```python
from build123d import *

# Parameters (mm, degrees)
SKETCH1_R               = 150
BOSS_EXTRUDE1_DEPTH     = 9.09
SKETCH2_R               = 146.82
CUT_EXTRUDE1_DEPTH      = 15
SKETCH5_R               = 90
BOSS_EXTRUDE2_DEPTH     = 15
CHAMFER1_SIZE           = 5
FILLET6_R               = 10
SKETCH6_R               = 1.55
CUT_EXTRUDE2_DEPTH      = 5
SKETCH7_R               = 16
CUT_EXTRUDE3_DEPTH      = 4.8
BOSS_EXTRUDE3_START     = 4.8
BOSS_EXTRUDE3_DEPTH     = 4.8
CIRPATTERN1_COUNT       = 30
SKETCH17_W              = 2.73
SKETCH17_H              = 90
SKETCH23_W              = 41
SKETCH23_H              = 20
CUT_EXTRUDE6_DEPTH      = 213.486594636
CUT_EXTRUDE7_DEPTH      = 213.486594636
CUT_EXTRUDE7_DEPTH_BACK = 213.486594636
SKETCH24_R              = 1.47
SKETCH26_R              = 150
SKETCH26_R_2            = 120
BOSS_EXTRUDE4_DEPTH     = 16.64


with BuildPart() as part:
    # Sketch1 → Boss-Extrude1 (new, symmetric)
    with BuildSketch(Plane.XY):
        Circle(SKETCH1_R)
    extrude(amount=BOSS_EXTRUDE1_DEPTH, both=True)

    # Sketch2 → Cut-Extrude1 (cut)
    with BuildSketch(Plane.XY.offset(9.09)):
        Circle(SKETCH2_R)
    extrude(amount=-CUT_EXTRUDE1_DEPTH, mode=Mode.SUBTRACT)

    # Sketch5 → Boss-Extrude2 (add)
    with BuildSketch(Plane.XY.offset(-5.91)):
        Circle(SKETCH5_R)
    extrude(amount=BOSS_EXTRUDE2_DEPTH)

    # Chamfer1
    chamfer1_edges = [part.edges().sort_by_distance(p)[0] for p in [
        (-90, 0, -5.91),
    ]]
    chamfer(chamfer1_edges, length=CHAMFER1_SIZE)

    # Fillet6
    fillet6_edges = [part.edges().sort_by_distance(p)[0] for p in [
        (-95, 0, -5.91),
    ]]
    fillet(fillet6_edges, radius=FILLET6_R)

    # Sketch6 → Cut-Extrude2 (cut)
    with BuildSketch(Plane.XY.offset(9.09)):
        with Locations((64.65, 0)):
            Circle(SKETCH6_R)
        with Locations((-68.33, 0)):
            Circle(SKETCH6_R)
        with Locations((-54.47, 24.14)):
            Circle(SKETCH6_R)
        with Locations((-54.47, -24.14)):
            Circle(SKETCH6_R)
        with Locations((50.79, -24.14)):
            Circle(SKETCH6_R)
        with Locations((50.79, 24.14)):
            Circle(SKETCH6_R)
    extrude(amount=-CUT_EXTRUDE2_DEPTH, mode=Mode.SUBTRACT)

    # Sketch7 → Cut-Extrude3 (cut)
    with BuildSketch(Plane.XY.offset(9.09)):
        Circle(SKETCH7_R)
    extrude(amount=-CUT_EXTRUDE3_DEPTH, mode=Mode.SUBTRACT)

    # Sketch8 → Boss-Extrude3 (add)
    with BuildSketch(Plane.XY.offset(4.29).offset(BOSS_EXTRUDE3_START)):
        with BuildLine():
            ThreePointArc((1.300521762, 15.947057507), (0.787845605, 15.007972717), (0.45011023, 13.992762443))
            ThreePointArc((0.45011023, 13.992762443), (0, 14), (-0.45011023, 13.992762443))
            ThreePointArc((-0.45011023, 13.992762443), (-0.787845605, 15.007972717), (-1.300521762, 15.947057507))
            ThreePointArc((-1.300521762, 15.947057507), (0, 16), (1.300521762, 15.947057507))
        make_face()
    boss_extrude3 = extrude(amount=-BOSS_EXTRUDE3_DEPTH)

    # CirPattern1: Boss-Extrude3 ×30 about axis
    cirpattern1_axis = Axis((0, 0, 0), (0, 0, 1))
    for i in range(1, CIRPATTERN1_COUNT):
        add(boss_extrude3.rotate(cirpattern1_axis, i * 360 / CIRPATTERN1_COUNT))

    # Sketch17 → Cut-Revolve4 (revolve, cut)
    with BuildSketch(Plane(origin=(0, 0, 0), x_dir=(0, 0, -1), z_dir=(1, 0, 0))):
        with Locations((-4.545, 45)):
            Rectangle(SKETCH17_W, SKETCH17_H)
    revolve(axis=Axis((0, 0, -0.91), (0, 0, 1)), mode=Mode.SUBTRACT)


with BuildPart() as cut_revolve4_piece_1:
    # of the separate pieces the step leaves, piece 1, a body of its own (cut_revolve4_pieces)
    add(part.part.solids().sort_by_distance((99.142135624, 0, -5.91))[0])

    # Sketch23 → Cut-Extrude6 (cut, through all)
    with BuildSketch(Plane.XY.offset(3.18)):
        with Locations((-10.44, 0)):
            Rectangle(SKETCH23_W, SKETCH23_H)
    extrude(amount=-CUT_EXTRUDE6_DEPTH, mode=Mode.SUBTRACT)

    # Sketch24 → Cut-Extrude7 (cut, two sides: drawn at the far end of the back side and taken through both)
    with BuildSketch(Plane.XY.offset(3.18).offset(-CUT_EXTRUDE7_DEPTH_BACK)):
        with Locations((-35.419501393, -5.08)):
            Circle(SKETCH24_R)
        with Locations((14.680498607, -5.08)):
            Circle(SKETCH24_R)
        with Locations((-35.419501393, 5.08)):
            Circle(SKETCH24_R)
        with Locations((14.680498607, 5.08)):
            Circle(SKETCH24_R)
    extrude(amount=CUT_EXTRUDE7_DEPTH + CUT_EXTRUDE7_DEPTH_BACK, mode=Mode.SUBTRACT)

    # Sketch26 → Boss-Extrude4 (add)
    with BuildSketch(Plane(origin=(0, 0, -9.09), x_dir=(-1, 0, 0), z_dir=(0, 0, -1))):
        Circle(SKETCH26_R)
        Circle(SKETCH26_R_2, mode=Mode.SUBTRACT)
    extrude(amount=BOSS_EXTRUDE4_DEPTH)


with BuildPart() as cut_revolve4_piece_2:
    # of the separate pieces the step leaves, piece 2, a body of its own (cut_revolve4_pieces)
    add(part.part.solids().sort_by_distance((90, 0, 5.91))[0])


solid = cut_revolve4_piece_1.part
```
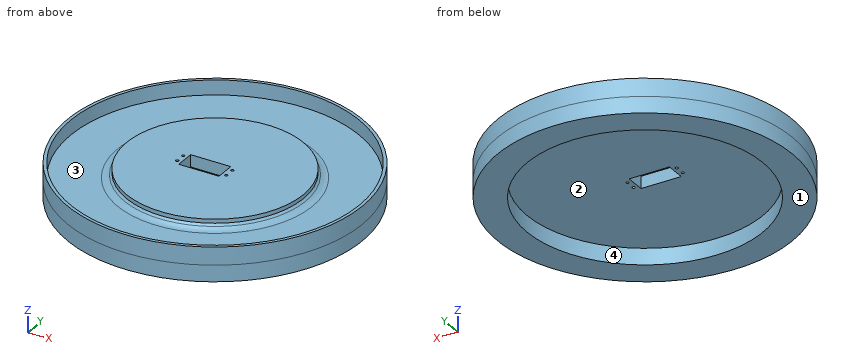
The listing builds one solid part. Answer for the finished solid, in the listing's coordinates (mm). Face numbers are marked on the shaded views. A direction names the side the tool comes from. Coordinates: 2 decimals unless noted, no trailing zeros. Write each loop counter-clockwise with the first axis right and the second up, starting at its lowest first coordinate (ties: lowest second). Pieces come first, ordered by that corner, then holes. Notation, with made-up numbers: (63, 46.25) - (119, 46.25) arc R21 ccw to (119, 70.25) - close; hole circle Ø6 at (-32, -10). An arc over 180 degrees is marked (long way). Return JSON: item names as keys, results as strings. Group by question number.
1. Given pin 1 (2 mm diameter, centred on x = -3, z = -6, fed in from +Y); pin 2 (5 mm diameter, centred on x = 59.5, z = -14.5, fed in from +Y); pin 3 (2.5 mm diameter, centred on x = 14.68, y = 5.08, fed in from -Z); pin 4 (13.5 mm diameter, centred on x = -16.5, z = -2.5, fed in from -Y), each flat-ended and moving along its own axis, determine where each tip first touches the part or whether it passes through.
2. Determine the mould class of the marked faces 1 and 2 for opening direction X: released by +X, released by -X, zero draft, split by the parting line, or undercut.
3. A cutting plane is placed at B-B, the plane x = 0. Determine the outline of the cut face in (y, z), plus the area to 3 significant figures.
4. A cutting plane is placed at C-C, the plane z = -21. Determine the outline of the cut face in (x, y), plus the area to 3 significant figures.
5. Straight lines are drawn through the part: L1, parallel to Y at x = 0, z = -15; L2, parallel to Y at x = -15, z = -5; L3, parallel to X at y = 5, z = -2. For each, find the intervals that lie inside material, in ascending order.
6. A cutting plane is placed at A-A, the plane y = 0. Determine the outline of the cut face in (x, z).
7. Which of the six approach directions +Z, -Z, +X, -X, +Y, -Y give full straight-line access (tool end or side, diameter ignored) to the marked faces 3 and 4?
Ans:
{
 "1": {"pin 1": "y = 149.99", "pin 2": "y = 138.75", "pin 3": "through", "pin 4": "y = -149.68"},
 "2": {"face 1": "zero draft", "face 2": "undercut"},
 "3": {"outline": "(-150, -25.73) - (-120, -25.73) - (-120, -9.09) - (-10, -9.09) - (-10, 3.18) - (-90, 3.18) - (-90, -0.91) - (-92.07, -2.98) arc R10 cw to (-99.14, -5.91) - (-146.82, -5.91) - (-146.82, 9.09) - (-150, 9.09) - close; (10, -9.09) - (120, -9.09) - (120, -25.73) - (150, -25.73) - (150, 9.09) - (146.82, 9.09) - (146.82, -5.91) - (99.14, -5.91) arc R10 cw to (92.07, -2.98) - (90, -0.91) - (90, 3.18) - (10, 3.18) - close", "area": "3,470 mm²"},
 "4": {"outline": "circle Ø300 at (0, 0); hole circle Ø240 at (0, 0)", "area": "25,400 mm²"},
 "5": {"L1": "-150 to -120, 120 to 150", "L2": "-149.25 to -146.05, -93.78 to -10, 10 to 93.78, 146.05 to 149.25", "L3": "-149.92 to -146.73, -90.95 to -36.89, -33.95 to -30.94, 10.06 to 13.21, 16.15 to 90.95, 146.73 to 149.92"},
 "6": {"outline": "(-150, -25.73) - (-120, -25.73) - (-120, -9.09) - (-30.94, -9.09) - (-30.94, 3.18) - (-90, 3.18) - (-90, -0.91) - (-92.07, -2.98) arc R10 cw to (-99.14, -5.91) - (-146.82, -5.91) - (-146.82, 9.09) - (-150, 9.09) - close; (10.06, -9.09) - (120, -9.09) - (120, -25.73) - (150, -25.73) - (150, 9.09) - (146.82, 9.09) - (146.82, -5.91) - (99.14, -5.91) arc R10 cw to (92.07, -2.98) - (90, -0.91) - (90, 3.18) - (10.06, 3.18) - close"},
 "7": {"face 3": "+Z", "face 4": "-Z"}
}
